```python
from build123d import *

# Parameters (mm, degrees)
F0_R     = 2.55
F0_W     = 7.4266694462
F0_H     = 7.0167635567
F0_W_2   = 8.4439013153
F0_H_2   = 2.6164194569
F0_H_3   = 1.3082097284
F1_DEPTH = 35
F2_T     = -1.2


with BuildPart() as f1:
    # F0 (on Top) → F1 (new body)
    with BuildSketch(Plane.XY):
        with BuildLine():
            Line((12.5671070093, 2.2891284898), (12.5671070093, -4.3818661943))
            Line((12.5671070093, -4.3818661943), (27.0671070093, -4.3818661943))
            Line((27.0671070093, -4.3818661943), (27.0671070093, -2.9131628679))
            ThreePointArc((27.0671070093, -2.9131628679), (25.1741554355, -3.3857602737), (23.5011908077, -2.3818661943))
            ThreePointArc((23.5011908077, -2.3818661943), (23.7463344607, 0.9390381298), (27.0671070093, 1.1859604264))
            ThreePointArc((27.0671070093, 1.1859604264), (27.8271392688, 0.2839446425), (28.0999395649, -0.8636012208))
            ThreePointArc((28.0999395649, -0.8636012208), (27.9713863773, -1.6630356049), (27.5986883221, -2.3818661943))
            Line((27.5986883221, -2.3818661943), (30.0671070093, -2.3818661943))
            Line((30.0671070093, -2.3818661943), (30.0671070093, 19.4367093172))
            Line((30.0671070093, 19.4367093172), (30.4183758122, 42.5877915199))
            ThreePointArc((30.4183758122, 42.5877915199), (29.8435067876, 44.0215787509), (28.418605989, 44.6181338057))
            Line((28.418605989, 44.6181338057), (25.8984067957, 44.6181338057))
            ThreePointArc((25.8984067957, 44.6181338057), (24.724883132, 44.2376529352), (23.9978627735, 43.2409760165))
            Line((23.9978627735, 43.2409760165), (18.2440858049, 25.6838704894))
            ThreePointArc((18.2440858049, 25.6838704894), (17.1535552671, 24.1888551114), (15.3932697716, 23.6181338057))
            Line((15.3932697716, 23.6181338057), (12.5671070093, 23.6181338057))
            Line((12.5671070093, 23.6181338057), (12.5671070093, 13.2305212319))
            Line((12.5671070093, 13.2305212319), (19.9937764555, 13.2305212319))
            Line((19.9937764555, 13.2305212319), (19.9937764555, 6.2137576751))
            Line((19.9937764555, 6.2137576751), (28.4376777709, 6.2137576751))
            Line((28.4376777709, 6.2137576751), (28.4376777709, 3.5973382182))
            Line((28.4376777709, 3.5973382182), (19.9937764555, 3.5973382182))
            Line((19.9937764555, 3.5973382182), (19.9937764555, 2.2891284898))
            Line((19.9937764555, 2.2891284898), (12.5671070093, 2.2891284898))
        make_face()
        with Locations((27.1516455619, 40.181864053)):
            Circle(F0_R, mode=Mode.SUBTRACT)
        with BuildLine():
            Line((-1.9328929907, -4.3818661943), (12.5671070093, -4.3818661943))
            Line((12.5671070093, -4.3818661943), (12.5671070093, 2.2891284898))
            Line((12.5671070093, 2.2891284898), (5.1404375632, 2.2891284898))
            Line((5.1404375632, 2.2891284898), (5.1404375632, 3.5973382182))
            Line((5.1404375632, 3.5973382182), (-3.3034637522, 3.5973382182))
            Line((-3.3034637522, 3.5973382182), (-3.3034637522, 6.2137576751))
            Line((-3.3034637522, 6.2137576751), (5.1404375632, 6.2137576751))
            Line((5.1404375632, 6.2137576751), (5.1404375632, 13.2305212319))
            Line((5.1404375632, 13.2305212319), (12.5671070093, 13.2305212319))
            Line((12.5671070093, 13.2305212319), (12.5671070093, 23.6181338057))
            Line((12.5671070093, 23.6181338057), (9.7409442471, 23.6181338057))
            ThreePointArc((9.7409442471, 23.6181338057), (7.9806587516, 24.1888551114), (6.8901282137, 25.6838704894))
            Line((6.8901282137, 25.6838704894), (1.1363512452, 43.2409760165))
            ThreePointArc((1.1363512452, 43.2409760165), (0.4093308866, 44.2376529352), (-0.764192777, 44.6181338057))
            Line((-0.764192777, 44.6181338057), (-2.0242923737, 44.6181338057))
            Line((-2.0242923737, 44.6181338057), (-3.2843919703, 44.6181338057))
            Line((-3.2843919703, 44.6181338057), (-3.2843919703, 42.6181338057))
            Line((-3.2843919703, 42.6181338057), (-5.2841617935, 42.5877915199))
            Line((-5.2841617935, 42.5877915199), (-4.9328929907, 19.4367093172))
            Line((-4.9328929907, 19.4367093172), (-4.9328929907, -2.3818661943))
            Line((-4.9328929907, -2.3818661943), (-2.4644743034, -2.3818661943))
            ThreePointArc((-2.4644743034, -2.3818661943), (-2.9378845991, -0.4878170914), (-1.9328929907, 1.1859604264))
            ThreePointArc((-1.9328929907, 1.1859604264), (0.7318203171, 1.4135984832), (2.1342744538, -0.8636012208))
            ThreePointArc((2.1342744538, -0.8636012208), (2.0057212662, -1.6630356049), (1.633023211, -2.3818661943))
            ThreePointArc((1.633023211, -2.3818661943), (-0.0399414169, -3.3857602737), (-1.9328929907, -2.9131628679))
            Line((-1.9328929907, -2.9131628679), (-1.9328929907, -4.3818661943))
        make_face()
        with BuildLine():
            ThreePointArc((0.5325684568, 40.181864053), (-3.8181265316, 38.3763177205), (-2.0242923737, 42.7318548234))
            ThreePointArc((-2.0242923737, 42.7318548234), (-0.2167365548, 41.9874103855), (0.5325684568, 40.181864053))
        make_face(mode=Mode.SUBTRACT)
        with BuildLine():
            Line((27.0671070093, -2.9131628679), (27.0671070093, -4.3818661943))
            Line((27.0671070093, -4.3818661943), (28.0671070093, -4.3818661943))
            ThreePointArc((28.0671070093, -4.3818661943), (29.4813205717, -3.7960797567), (30.0671070093, -2.3818661943))
            Line((30.0671070093, -2.3818661943), (27.5986883221, -2.3818661943))
            ThreePointArc((27.5986883221, -2.3818661943), (27.3525789154, -2.6672063249), (27.0671070093, -2.9131628679))
        make_face()
        with BuildLine():
            Line((-2.9328929907, -4.3818661943), (-1.9328929907, -4.3818661943))
            Line((-1.9328929907, -4.3818661943), (-1.9328929907, -2.9131628679))
            ThreePointArc((-1.9328929907, -2.9131628679), (-2.2183648967, -2.6672063249), (-2.4644743034, -2.3818661943))
            Line((-2.4644743034, -2.3818661943), (-4.9328929907, -2.3818661943))
            ThreePointArc((-4.9328929907, -2.3818661943), (-4.347106553, -3.7960797567), (-2.9328929907, -4.3818661943))
        make_face()
        with BuildLine():
            ThreePointArc((-3.2843919703, 44.6181338057), (-4.7092927689, 44.0215787509), (-5.2841617935, 42.5877915199))
            Line((-5.2841617935, 42.5877915199), (-3.2843919703, 42.6181338057))
            Line((-3.2843919703, 42.6181338057), (-3.2843919703, 44.6181338057))
        make_face()
        with Locations((8.8537722862, 9.7221394535)):
            Rectangle(F0_W, F0_H)
        with Locations((16.2804417324, 9.7221394535)):
            Rectangle(F0_W, F0_H)
        with Locations((24.2157271132, 4.9055479467)):
            Rectangle(F0_W_2, F0_H_2)
        with Locations((8.8537722862, 4.9055479467)):
            Rectangle(F0_W, F0_H_2)
        with Locations((0.9184869055, 4.9055479467)):
            Rectangle(F0_W_2, F0_H_2)
        with Locations((8.8537722862, 2.943233354)):
            Rectangle(F0_W, F0_H_3)
        with Locations((16.2804417324, 4.9055479467)):
            Rectangle(F0_W, F0_H_2)
        with Locations((16.2804417324, 2.943233354)):
            Rectangle(F0_W, F0_H_3)
    extrude(amount=F1_DEPTH)

    # F2
    f2_openings = [f1.faces().sort_by_distance(p)[0] for p in [
        (12.567107, 16.00407, 35),
    ]]
    offset(amount=F2_T, openings=f2_openings)


solid = f1.part
```
Part model, mm, in its own coordinate system. A direction names the side the tool comes from. Round coordinates to 2 decimals unless told otherwise and drop trailing zeros. Write each loop counter-clockwise with the first axis right and the second up, starting at its lowest first coordinate (ties: lowest second). Pieces come first, ordered by that corner, then holes. Notation, with made-up numbers: M 22.25,-17 L 44.25,-17 A20 ccw 44.25,2 Z; hole C -5.5,73 d9. An arc over 180 degrees is marked long. Answer as CSV lines item,"result". Start each with the question number.
1) Band-saw the part on C-C (z = 28). Count the separate pieces of the cut face and the enclosed holes in it, then the cut area to 3 significant figures.
2) Band-saw the part on A-A (y = 35). List the corners of the cut face in (x, z).
3) Drill centre lines: L1, parallel to X at y = 5, z = 30.5; L2, parallel to X at y = 41, z = 28.5; L3, parallel to X at y = 42, z = 12. Where is each one in solid material? Low to high.
4) Which spindle directions (+Z, -Z, +X, -X, +Y, -Y) get a long thin tool onto all of the face, cutting with end or side? Do faces 1 (the face through (7, 24, 35)), 2 (the face through (17.17, 24.2, 17.26)), 3 (the face through (12, -3.182, 18)), 4 (the face through (30.067, 8, 17)), 5 (the face through (-4.363, -3.78, 17.255)). Say none if no direction does.
5) Drop flat-ended pins along their axis: pin 1 (8 mm diameter, centred on y = 17, z = 26, fed in from -X); pin 2 (10 mm diameter, centred on y = 29, z = 9, fed in from -X); pin 3 (9.5 mm diameter, centred on y = 7.5, z = 15.5, fed in from +X); pin 4 (4 mm diameter, centred on x = 27.15, y = 40.18, fed in from -Z). Give the stop position or say it passes through.
6) Band-saw the part on D-D (y = 16). List the corners of the cut face in (x, z).
7) Mould opens along Y. For faces 6 (the face through (29.47, -3.81, 17.26)), 7 (the face through (21.595, 32.056, 17.863)), 8 (the face through (12, 15, 0)), 9 (the face through (3.6, 31.87, 17.86)) say: +Y half, -Y half, draft (parallel to the pull), parting line (faces both ways), or undercut.
8) Band-saw the part on B-B (x = 26.5). List the corners of the cut face in (y, z), then the cut area to 3 significant figures.
Worked out:
1,separate pieces,"1"
1,enclosed holes,"5"
1,area,"284 mm²"
2,outline,"M -5.17,0 L 3.84,0 L 3.84,35 L 2.57,35 L 2.57,1.2 L -3.97,1.2 L -3.97,35 L -5.17,35 Z; M 21.3,0 L 30.3,0 L 30.3,35 L 29.1,35 L 29.1,1.2 L 22.56,1.2 L 22.56,35 L 21.3,35 Z"
3,L1,"-4.93 to -3.73, 28.87 to 30.07"
3,L2,"-5.26 to -4.43, 0.4 to 1.87, 23.26 to 24.74, 29.57 to 30.39"
3,L3,"-5.28 to -3.81, -0.23 to 1.54, 23.59 to 25.36, 28.94 to 30.41"
4,face 1,"+Z, +X, -X, +Y, -Y"
4,face 2,"+Z, -Z, +Y"
4,face 3,"+Z"
4,face 4,"+Z, -Z, +X, -Y"
4,face 5,"+Z, -Z, -X, -Y"
5,pin 1,"x = -4.96"
5,pin 2,"x = -5.15"
5,pin 3,"x = 30.07"
5,pin 4,"through"
6,outline,"M -4.93,0 L 30.07,0 L 30.07,35 L 28.87,35 L 28.87,1.2 L -3.73,1.2 L -3.73,35 L -4.93,35 Z"
7,face 6,"-Y half"
7,face 7,"undercut"
7,face 8,"draft"
7,face 9,"undercut"
8,outline,"M -4.38,0 L -3.23,0 L -3.23,35 L -4.38,35 Z; M 1.5,0 L 37.72,0 L 37.72,35 L 36.49,35 L 36.49,1.2 L 2.76,1.2 L 2.76,35 L 1.5,35 Z; M 42.65,0 L 44.62,0 L 44.62,35 L 42.65,35 Z"
8,area,"237 mm²"
